```python
from build123d import *

# Parameters (mm, degrees)
SKETCH1_W           = 8
SKETCH1_H           = 38.25
SKETCH2_R           = 3
BOSS_EXTRUDE1_DEPTH = 2
BOSS_EXTRUDE2_DEPTH = 8
CUT_EXTRUDE1_DEPTH  = 2
CUT_EXTRUDE2_DEPTH  = 26.5
CUT_EXTRUDE3_DEPTH  = 26.5
SKETCH7_W           = 0.25
SKETCH7_H           = 2
BOSS_EXTRUDE3_DEPTH = 3.5
SKETCH8_W           = 0.25
SKETCH8_H           = 2
BOSS_EXTRUDE4_DEPTH = 3.5
SKETCH9_R           = 2.95
BOSS_EXTRUDE5_DEPTH = 1
FILLET1_R           = 0.5


with BuildPart() as part:
    # Sketch1 → Revolve1 (revolve)
    with BuildSketch(Plane.XZ):
        with Locations((4, 19.125)):
            Rectangle(SKETCH1_W, SKETCH1_H)
    revolve(axis=Axis((0, 0, 38.25), (0, 0, -1)))

    # Sketch2 → Boss-Extrude1 (add)
    with BuildSketch(Plane(origin=(0, 0, 0), x_dir=(-1, 0, 0), z_dir=(0, 0, -1))):
        Circle(SKETCH2_R)
    extrude(amount=BOSS_EXTRUDE1_DEPTH)

    # Sketch3 → Boss-Extrude2 (add)
    with BuildSketch(Plane(origin=(0, 0, -2), x_dir=(-1, 0, 0), z_dir=(0, 0, -1))):
        with BuildLine():
            Line((-1, -1.118033989), (-1, 1.118033989))
            ThreePointArc((-1, 1.118033989), (1.5, 0), (-1, -1.118033989))
        make_face()
    extrude(amount=BOSS_EXTRUDE2_DEPTH)

    # Sketch4 → Cut-Extrude1 (cut)
    with BuildSketch(Plane(origin=(0, 0, -2), x_dir=(-1, 0, 0), z_dir=(0, 0, -1))):
        with BuildLine():
            Line((-1, -1.118033989), (-1, 1.118033989))
            ThreePointArc((-1, 1.118033989), (-1.5, 0), (-1, -1.118033989))
        make_face()
    extrude(amount=-CUT_EXTRUDE1_DEPTH, mode=Mode.SUBTRACT)

    # Sketch5 → Cut-Extrude2 (cut)
    with BuildSketch(Plane.XY.offset(38.25)):
        with BuildLine():
            Line((-5.402777064, 5.9), (5.402777064, 5.9))
            ThreePointArc((5.402777064, 5.9), (0, 8), (-5.402777064, 5.9))
        make_face()
    extrude(amount=-CUT_EXTRUDE2_DEPTH, mode=Mode.SUBTRACT)

    # Sketch6 → Cut-Extrude3 (cut)
    with BuildSketch(Plane.XY.offset(38.25)):
        with BuildLine():
            Line((5.402777064, -5.9), (-5.402777064, -5.9))
            ThreePointArc((-5.402777064, -5.9), (0, -8), (5.402777064, -5.9))
        make_face()
    extrude(amount=-CUT_EXTRUDE3_DEPTH, mode=Mode.SUBTRACT)

    # Sketch7 → Boss-Extrude3 (add)
    with BuildSketch(Plane.XY.offset(38.25)):
        with Locations((-6.375, 0)):
            Rectangle(SKETCH7_W, SKETCH7_H)
    extrude(amount=BOSS_EXTRUDE3_DEPTH)

    # Sketch8 → Boss-Extrude4 (add)
    with BuildSketch(Plane.XY.offset(38.25)):
        with Locations((6.375, 0)):
            Rectangle(SKETCH8_W, SKETCH8_H)
    extrude(amount=BOSS_EXTRUDE4_DEPTH)

    # Sketch9 → Boss-Extrude5 (add)
    with BuildSketch(Plane.XY.offset(38.25)):
        Circle(SKETCH9_R)
    extrude(amount=BOSS_EXTRUDE5_DEPTH)

    # Fillet1
    fillet1_edges = [part.edges().sort_by_distance(p)[0] for p in [
        (0, 8, 11.75),
        (0, -8, 11.75),
        (-8, 0, 0),
        (-6.375, -1, 41.75),
        (-6.375, 1, 41.75),
        (6.375, -1, 41.75),
        (6.375, 1, 41.75),
        (-2.95, 0, 39.25),
    ]]
    fillet(fillet1_edges, radius=FILLET1_R)


solid = part.part
```
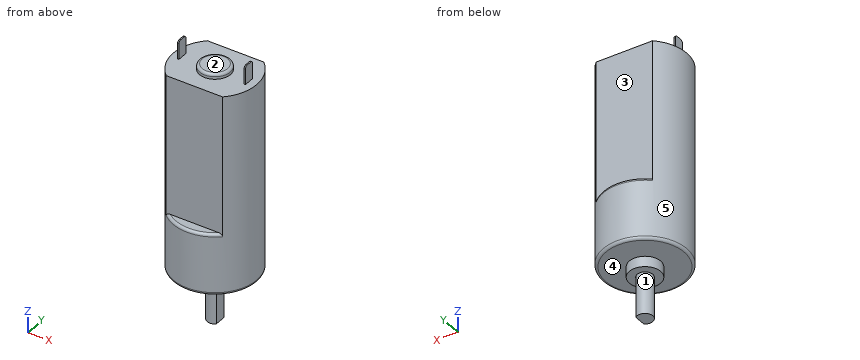
Can you work these out from the model? Positions are in its coordinate system, mm. Face numbers are marked on the shaded views. A direction names the side the tool comes from. Coordinates: 2 decimals unless noted, no trailing zeros. Loops run counter-clockwise (first coordinate to the right, second up) from the corner with the lowest first, then second, coordinate; pieces in that order, holes last. Notation, with made-up numbers: (75, 42) -> (130, 42) arc R35 ccw to (130, 74) -> close; hole circle Ø5 at (62, -27.5). An arc over 180 degrees is marked (long way). Answer as a JSON object with one key per item and string values.
1) If I drill on line 1 (Z direction, x = -1.25, y = -1.5); line 2 (Z direction, x = 3, y = -2.25); line 3 (Y direction, x = -0.5, z = 37), over which ranges is the centre line in solid material (lowest first)?
Results:
{"line 1": "z = -2 to 39.25", "line 2": "z = 0 to 38.25", "line 3": "y = -5.9 to 5.9"}
2) Imagine slicing it at B-B (z = 10). Please give me the cut outline in (x, y), then the cut area to 3 significant figures.
Results:
{"outline": "circle Ø16 at (0, 0)", "area": "201 mm^2"}
3) Imagine slicing it at D-D (z = -6). Please give me the cut outline in (x, y), then the cut area to 3 significant figures.
Results:
{"outline": "(1, -1.12) -> (1, 1.12) arc R1.5 ccw (long way) to start", "area": "6.29 mm^2"}
4) Imagine slicing it at A-A (x = 0). Please give me the cut outline in (y, z), then the cut area to 3 significant figures.
Results:
{"outline": "(-8, 0.5) arc R0.5 ccw to (-7.5, 0) -> (-3, 0) -> (-3, -2) -> (-1.5, -2) -> (-1.5, -10) -> (1.5, -10) -> (1.5, -2) -> (3, -2) -> (3, 0) -> (7.5, 0) arc R0.5 ccw to (8, 0.5) -> (8, 11.25) arc R0.5 ccw to (7.5, 11.75) -> (5.9, 11.75) -> (5.9, 38.25) -> (2.95, 38.25) -> (2.95, 38.75) arc R0.5 ccw to (2.45, 39.25) -> (-2.45, 39.25) arc R0.5 ccw to (-2.95, 38.75) -> (-2.95, 38.25) -> (-5.9, 38.25) -> (-5.9, 11.75) -> (-7.5, 11.75) arc R0.5 ccw to (-8, 11.25) -> close", "area": "542 mm^2"}
5) For the marked faces 4 and 5, which set-ups out of +Z, -Z, +X, -X, +Y, -Y let a thin tool reach every point of the face, with its end or its side?
Results:
{"face 4": "-Z", "face 5": "+Z, -Z"}
6) Imagine slicing it at C-C (z = 22.5). Please give me the cut outline in (x, y).
Results:
{"outline": "(-5.4, -5.9) -> (5.4, -5.9) arc R8 ccw to (5.4, 5.9) -> (-5.4, 5.9) arc R8 ccw to start"}
7) Thinking about a two-plate mould opening in X: for the marked faces 1, 2 and 3, which applies, pulls with the +X half, pulls with the -X half, needs draft (parallel to the pull), parting line crosses it, or undercut?
Results:
{"face 1": "parting line crosses it", "face 2": "undercut", "face 3": "needs draft"}
8) For P1, Ø1.5, axis at x = 6, y = 5, coming from the -Z side; P2, Ø3, axis at x = -2.5, z = 20.5, coming from the -Y side; P3, Ø1.5, axis at x = -0.5, y = -1, coming from the +Z side, each with a flat end and sliding along its axis, tell me the tip position at first contact or that it passes through.
Results:
{"P1": "stops at z = 0", "P2": "stops at y = -5.9", "P3": "stops at z = 39.25"}
